Can you work these out from the model? Positions are in its coordinate system, mm. Face numbers are marked on the shaded views. A direction names the side the tool comes from. Coordinates: 2 decimals unless noted, no trailing zeros. Order: outer loops, then holes, each group sorted by start corner. A loop starts at its lowest first (then second) coordinate and runs counter-clockwise, first axis right, second up. Notation, with made-up numbers: (40.5, 6) -> (51.5, 6) arc R16 cw to (51.5, 19) -> close; hole circle Ø1 at (55.5, 54.25). An arc over 180 degrees is marked (long way). Answer in a Markdown table with one row per item. Add a question column.
1. We'd pull the mould along Y, two halves only. Please class the marked faces 1, 2 and 3: pulls with the +Y half, pulls with the -Y half, needs draft (parallel to the pull), parting line crosses it, or undercut.
2. Imagine slicing it at C-C on x = 47. Write out the boundary of the cut face in (y, z), plus the area to 3 significant figures.
3. Will these pins go through, and if not, where does the flat tip stop? pin 1 (2 mm diameter, centred on y = -64, z = 37, fed in from -X); pin 2 (20 mm diameter, centred on x = -8.5, z = 12.5, fed in from -Y); pin 3 (7.5 mm diameter, centred on x = -16.5, z = 11, fed in from +Y).
4. On a 3-axis mill with a long thin cutter (end or side, diameter ignored), from which of +Z, -Z, +X, -X, +Y, -Y can I reach the whole of each face in a straight line? I mean the marked faces 4, 5 and 6. Say none if no direction works.
5. If I drill on line 1 along Z through (x, y) = (110, -88); line 2 along Z through (x, y) = (115, 44); line 3 along Y through (x, z) = (9.5, 12), over which ranges is the centre line in solid material (lowest first)? Write a range as [from, to].
6. Imagine slicing it at D-D on y = -6. Write out the boundary of the cut face in (x, z), plus the area to 3 significant figures.
7. Imagine slicing it at B-B on z = 37. Write out the boundary of the cut face in (x, y).
8. Imagine slicing it at A-A on y = 90. Write out the boundary of the cut face in (x, z), plus the area to 3 significant figures.
from build123d import *

# Parameters (mm, degrees)
BOSS_EXTRUDE4_DEPTH = 20
SKETCH1_5_R         = 30
SKETCH1_5_R_2       = 15
SKETCH1_5_R_3       = 17.5
BOSS_EXTRUDE5_DEPTH = 25
SKETCH1_6_R         = 15
SKETCH1_6_R_2       = 17.5
BOSS_EXTRUDE6_DEPTH = 43


with BuildPart() as part:
    # Sketch1 → Boss-Extrude4 (new body)
    with BuildSketch(Plane.XY):
        with BuildLine():
            Line((-130, 60), (-35, 42.5))
            Line((-35, 42.5), (-35, 50))
            ThreePointArc((-35, 50), (-33.535533906, 53.535533906), (-30, 55))
            Line((-30, 55), (0, 55))
            ThreePointArc((0, 55), (54.567759373, 6.881833839), (13.655500107, -53.277831382))
            ThreePointArc((13.655500107, -53.277831382), (60.158955917, -61.243831597), (91.746142625, -96.2906317))
            ThreePointArc((91.746142625, -96.2906317), (107.681504867, -44.468355165), (161.565293978, -50.47013708))
            Line((161.565293978, -50.47013708), (112.993286108, 58.624378777))
            ThreePointArc((112.993286108, 58.624378777), (66.508772404, 114.25478106), (-4.020798406, 131.02175198))
            Line((-4.020798406, 131.02175198), (-130, 120))
            ThreePointArc((-130, 120), (-108.786796564, 111.213203436), (-100, 90))
            ThreePointArc((-100, 90), (-108.786796564, 68.786796564), (-130, 60))
        make_face()
        with BuildLine():
            ThreePointArc((0, 106), (84.0970935, 64.526574873), (102.386743403, -27.440021418))
            ThreePointArc((102.386743403, -27.440021418), (82.790250599, -38.752734171), (71.477537847, -19.156241367))
            ThreePointArc((71.477537847, -19.156241367), (58.709291689, 45.046854157), (0, 74))
            ThreePointArc((0, 74), (-16, 90), (0, 106))
        make_face(mode=Mode.SUBTRACT)
    extrude(amount=BOSS_EXTRUDE4_DEPTH)

    # Sketch1_5 → Boss-Extrude5 (add)
    # profile 1 of 3: a face of its own
    with BuildSketch(Plane.XY):
        with Locations(Location((-130, 90, 0), (0, 0, 90))):
            Circle(SKETCH1_5_R)
        with Locations((-130, 90)):
            Circle(SKETCH1_5_R_2, mode=Mode.SUBTRACT)
    # profile 2 of 3: a face of its own
    with BuildSketch(Plane.XY):
        with BuildLine():
            ThreePointArc((173.5, -80), (170.403521378, -64.074784052), (161.565293978, -50.47013708))
            ThreePointArc((161.565293978, -50.47013708), (107.681504867, -44.468355165), (91.746142625, -96.2906317))
            ThreePointArc((91.746142625, -96.2906317), (91.811890227, -96.446774947), (91.877270231, -96.60307247))
            ThreePointArc((91.877270231, -96.60307247), (139.471540144, -121.647124842), (173.5, -80))
        make_face()
        with Locations((131, -80)):
            Circle(SKETCH1_5_R_3, mode=Mode.SUBTRACT)
    # profile 3 of 3: a face of its own
    with BuildSketch(Plane.XY):
        with BuildLine():
            Line((-35, 50), (-35, 42.5))
            Line((-35, 42.5), (-35, 35))
            ThreePointArc((-35, 35), (-33.535533906, 31.464466094), (-30, 30))
            Line((-30, 30), (0, 30))
            ThreePointArc((0, 30), (30, 0), (0, -30))
            Line((0, -30), (-30, -30))
            ThreePointArc((-30, -30), (-33.535533906, -31.464466094), (-35, -35))
            Line((-35, -35), (-35, -50))
            ThreePointArc((-35, -50), (-33.535533906, -53.535533906), (-30, -55))
            Line((-30, -55), (0, -55))
            ThreePointArc((0, -55), (4.190718653, -54.840111936), (8.357072001, -54.361377352))
            ThreePointArc((8.357072001, -54.361377352), (10.996109007, -53.769839654), (13.655500107, -53.277831382))
            ThreePointArc((13.655500107, -53.277831382), (54.567759373, 6.881833839), (0, 55))
            Line((0, 55), (-30, 55))
            ThreePointArc((-30, 55), (-33.535533906, 53.535533906), (-35, 50))
        make_face()
    extrude(amount=BOSS_EXTRUDE5_DEPTH)

    # Sketch1_6 → Boss-Extrude6 (add)
    with BuildSketch(Plane.XY):
        with Locations((-130, 90)):
            Circle(SKETCH1_6_R)
        with Locations((131, -80)):
            Circle(SKETCH1_6_R_2)
    extrude(amount=BOSS_EXTRUDE6_DEPTH)


solid = part.part
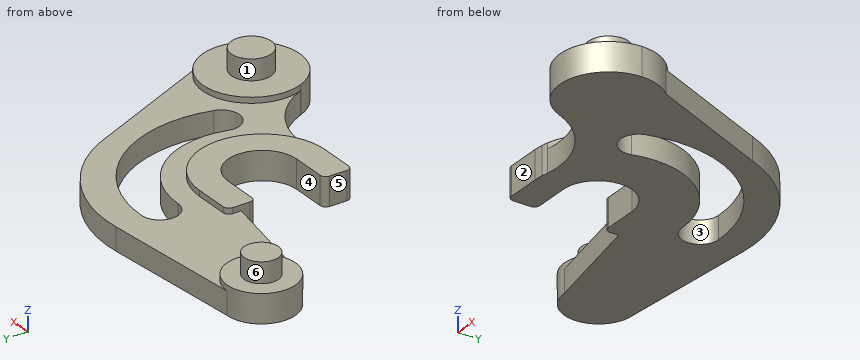
Answers follow:
| question | item | result |
|---|---|---|
| 1 | face 1 | parting line crosses it |
| 1 | face 2 | pulls with the -Y half |
| 1 | face 3 | undercut |
| 2 | outline | (-55.62, 0) -> (57.16, 0) -> (57.16, 20) -> (28.57, 20) -> (28.57, 25) -> (-28.57, 25) -> (-28.57, 20) -> (-55.62, 20) -> close; (95.01, 0) -> (123.9, 0) -> (123.9, 20) -> (95.01, 20) -> close |
| 2 | area | 3,120 mm² |
| 3 | pin 1 | stops at x = 121.99 |
| 3 | pin 2 | stops at y = -55 |
| 3 | pin 3 | stops at y = 130.26 |
| 4 | face 4 | +Z, -Z, -X |
| 4 | face 5 | +Z, -Z, -X, -Y |
| 4 | face 6 | +Z |
| 5 | line 1 | z = [0, 25] |
| 5 | line 2 | z = [0, 20] |
| 5 | line 3 | y = [-54.09, -28.46], [28.46, 73.39], [105.57, 131.41] |
| 6 | outline | (29.39, 0) -> (73.76, 0) -> (73.76, 20) -> (54.67, 20) -> (54.67, 25) -> (29.39, 25) -> close; (105.83, 0) -> (141.77, 0) -> (141.77, 20) -> (105.83, 20) -> close |
| 6 | area | 1,730 mm² |
| 7 | outline | circle Ø30 at (-130, 90); circle Ø35 at (131, -80) |
| 8 | outline | (-160, 0) -> (-16, 0) -> (-16, 20) -> (-100, 20) -> (-100, 25) -> (-115, 25) -> (-115, 43) -> (-145, 43) -> (-145, 25) -> (-160, 25) -> close; (56, 0) -> (94.41, 0) -> (94.41, 20) -> (56, 20) -> close |
| 8 | area | 4,490 mm² |
